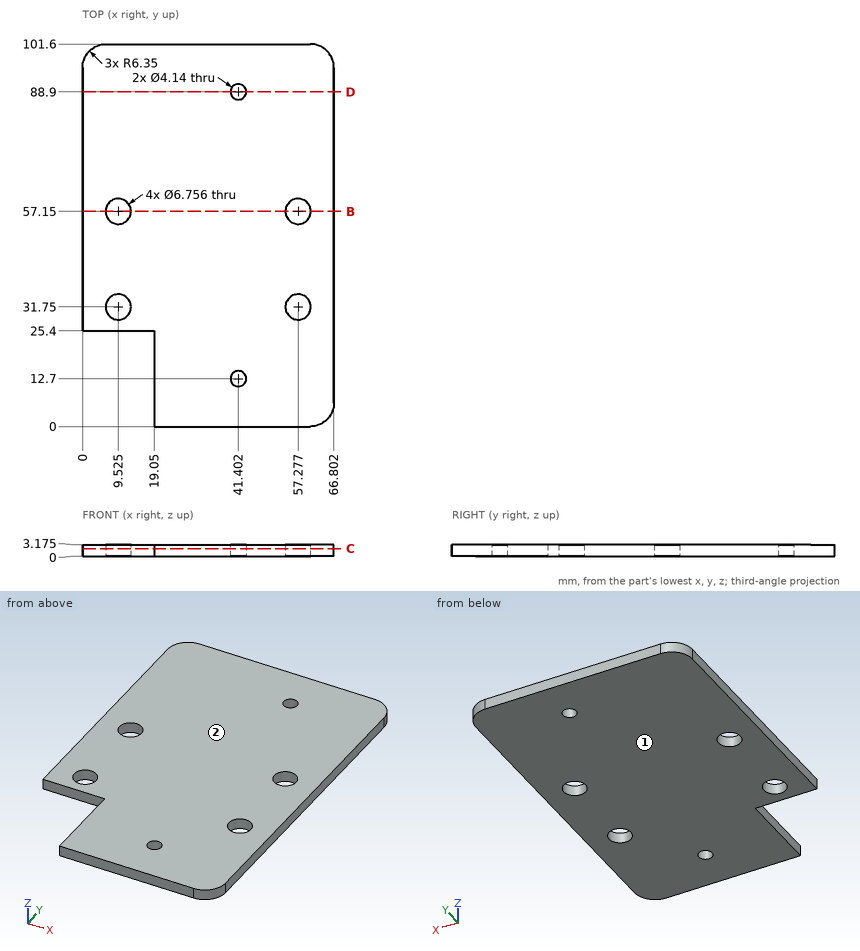
Drawing for the job (mm, zero at the part's lowest x, y, z). Round coordinates to 2 decimals unless told otherwise and drop trailing zeros. Write each loop counter-clockwise with the first axis right and the second up, starting at its lowest first coordinate (ties: lowest second). Pieces come first, ordered by that corner, then holes. Notation, with made-up numbers: (60.25, 59.5) - (93.25, 59.5) arc R21 cw to (93.25, 93.5) - close; hole circle Ø1 at (-13, 22). An arc over 180 degrees is marked (long way). Use CSV: the item, a comma, the result in double quotes.
(1) Band-saw the part on C-C (z = 2.1). Give the number of separate pieces and of enclosed holes in the cut face, plus the area to 3 significant figures.
Response:
separate pieces,"1"
enclosed holes,"6"
area,"6,110 mm²"
(2) Band-saw the part on D-D (y = 88.9). Write the cut outline in (x, z) (1 decimal).
Response:
outline,"(0, 0) - (39.3, 0) - (39.3, 3.2) - (0, 3.2) - close; (43.5, 0) - (66.8, 0) - (66.8, 3.2) - (43.5, 3.2) - close"
(3) Pin check, flat tip, straight feed: P1, Ø1, axis at x = 7, z = 2, coming from the -Y side. Stop position of the tip, or through.
Response:
P1,"y = 25.4"
(4) Mould opens along Z. For the marked faces 1 and 2 say: pulls with the +Z half, pulls with the -Z half, needs draft (parallel to the pull), parting line crosses it, or undercut.
Response:
face 1,"pulls with the -Z half"
face 2,"pulls with the +Z half"
(5) Wall check: line 1 (Y direction, x = 42, z = 2.9); line 2 (X direction, y = 34, z = 1.55) (1 decimal); line 3 (Y direction, x = 55, z = 2.5) (1 decimal). Give the ranges that are in metal, low to high.
Response:
line 1,"0 to 10.72, 14.68 to 86.92, 90.88 to 101.6"
line 2,"0 to 7, 12 to 54.8, 59.8 to 66.8"
line 3,"0 to 29.3, 34.2 to 54.7, 59.6 to 101.6"
(6) Band-saw the part on B-B (y = 57.15). Write the cut outline in (x, z) (1 decimal).
Response:
outline,"(0, 0) - (6.1, 0) - (6.1, 3.2) - (0, 3.2) - close; (12.9, 0) - (53.9, 0) - (53.9, 3.2) - (12.9, 3.2) - close; (60.7, 0) - (66.8, 0) - (66.8, 3.2) - (60.7, 3.2) - close"
